The listing builds one solid part. Answer for the finished solid, in the listing's coordinates (mm). Face numbers are marked on the shaded views. Coordinates: 2 decimals unless noted, no trailing zeros. Write each loop counter-clockwise with the first axis right and the second up, starting at its lowest first coordinate (ties: lowest second). Pieces come first, ordered by that corner, then holes.
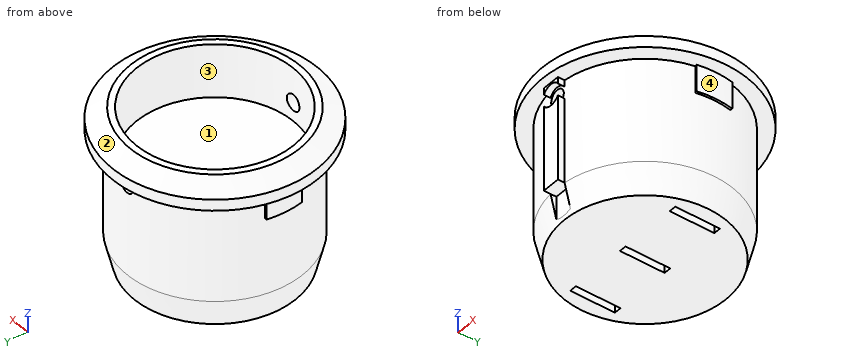
```python
from build123d import *

# Parameters (mm, degrees)
F0_R           = 11.5
F1_DEPTH       = 2.5
F2_R           = 9.85
F3_DEPTH       = 14.8
F4_SIZE2       = 3.2
F4_SIZE        = 0.8
F5_SIZE2       = 1.25
F5_SIZE        = 2
F6_R           = 8.8
F7_DEPTH       = 6
F8_W           = 0.8
F8_H           = 5
F9_DEPTH       = 5
F11_DEPTH      = 11.6
F12_W          = 2
F12_H          = 1.4
F13_DEPTH      = 3.2
F14_R          = 0.9
F15_DEPTH      = 22.0501071022
F17_END_RADIUS = 9.85
F16_R          = 1.2
F17_REACH      = 25.4442196519
F19_DEPTH      = 3


with BuildPart() as f1:
    # F0 (on Top) → F1 (new body)
    with BuildSketch(Plane.XY):
        Circle(F0_R)
    extrude(amount=F1_DEPTH)

    # F2 (on face) → F3 (join)
    with BuildSketch(Plane(origin=(0, 0, 0), x_dir=(1, 0, 0), z_dir=(0, 0, -1))):
        Circle(F2_R)
    extrude(amount=F3_DEPTH)

    # F4
    f4_edges = [f1.edges().sort_by_distance(p)[0] for p in [
        (-9.85, 0, -14.8),
    ]]
    f4_side = f1.faces().sort_by_distance((0, 0, -14.8))[0]
    chamfer(f4_edges, length=F4_SIZE, length2=F4_SIZE2, reference=f4_side)

    # F5
    f5_edges = [f1.edges().sort_by_distance(p)[0] for p in [
        (-11.5, 0, 2.5),
    ]]
    f5_side = f1.faces().sort_by_distance((0, 0, 2.5))[0]
    chamfer(f5_edges, length=F5_SIZE, length2=F5_SIZE2, reference=f5_side)

    # F6 (on face) → F7 (cut)
    with BuildSketch(Plane.XY.offset(2.5)):
        Circle(F6_R)
    extrude(amount=-F7_DEPTH, mode=Mode.SUBTRACT)

    # F8 (on face) → F9 (cut)
    with BuildSketch(Plane(origin=(0, 0, -14.8), x_dir=(1, 0, 0), z_dir=(0, 0, -1))):
        with Locations((-7.1, 0)):
            Rectangle(F8_W, F8_H)
        Rectangle(F8_W, F8_H)
        with Locations((7.1, 0)):
            Rectangle(F8_W, F8_H)
    extrude(amount=-F9_DEPTH, mode=Mode.SUBTRACT)

    # F10 (on face) → F11 (join)
    with BuildSketch(Plane(origin=(0, 0, 0), x_dir=(1, 0, 0), z_dir=(0, 0, -1))):
        with BuildLine():
            Line((-1, 10.5491071022), (-1, 9.7991071022))
            ThreePointArc((-1, 9.7991071022), (0, 9.85), (1, 9.7991071022))
            Line((1, 9.7991071022), (1, 10.5491071022))
            Line((1, 10.5491071022), (-1, 10.5491071022))
        make_face()
    extrude(amount=F11_DEPTH)

    # F12 (on face) → F13 (cut, through all)
    with BuildSketch(Plane(origin=(0, 0, -14.8), x_dir=(1, 0, 0), z_dir=(0, 0, -1))):
        with Locations((0, 9.8491071022)):
            Rectangle(F12_W, F12_H)
    extrude(amount=-F13_DEPTH, mode=Mode.SUBTRACT)

    # F14 (on face) → F15 (cut, through all)
    with BuildSketch(Plane.XZ.offset(10.5491071022)):
        with Locations((0, -1.4)):
            Circle(F14_R)
    extrude(amount=-F15_DEPTH, mode=Mode.SUBTRACT)

    f17_end = (Plane.XY.offset(-5.8) * Cylinder(F17_END_RADIUS, 124.5712732194, mode=Mode.PRIVATE)).faces().sort_by_distance((0, 9.85, -5.8))[0]
    # F16 (on face) → F17 (cut, up to the whole of a round face its end follows)
    with BuildSketch(Plane.XZ.offset(10.5491071022)):
        with Locations((0, -1.4)):
            Circle(F16_R)
    f17_long = extrude(amount=-F17_REACH, mode=Mode.PRIVATE)
    add(split(f17_long, bisect_by=f17_end, keep=Keep.ALL, mode=Mode.PRIVATE).solids().sort_by_distance((0, -10.5491071022, -1.4))[0], mode=Mode.SUBTRACT)

    # F18 (on face) → F19 (join)
    with BuildSketch(Plane(origin=(0, 0, 0), x_dir=(1, 0, 0), z_dir=(0, 0, -1))):
        with BuildLine():
            Line((-9.654950495, 1.9504950495), (-9.9, 2))
            ThreePointArc((-9.9, 2), (-10.1, 0), (-9.9, -2))
            Line((-9.9, -2), (-9.654950495, -1.9504950495))
            ThreePointArc((-9.654950495, -1.9504950495), (-9.85, 0), (-9.654950495, 1.9504950495))
        make_face()
        with BuildLine():
            Line((9.654950495, -1.9504950495), (9.9, -2))
            ThreePointArc((9.9, -2), (10.1, 0), (9.9, 2))
            Line((9.9, 2), (9.654950495, 1.9504950495))
            ThreePointArc((9.654950495, 1.9504950495), (9.85, 0), (9.654950495, -1.9504950495))
        make_face()
    extrude(amount=F19_DEPTH)


solid = f1.part
```
(1) Section B-B, the plane z = -10.5 is taken. Write down the section's boundary in (x, y), plus the area to 3 significant figures.
(2) For a pull along X with two mould halves and no side action, classify the marked faces 1, 2, 3 and 4 as pulls with the +X half, pulls with the -X half, needs draft (parallel to the pull), parting line crosses it, or undercut.
(3) Find the intervals of material crossed by probe 1 along Y at (x, z) = (0, 1); probe 2 along Z at (x, y) = (-5.25, 2.75); probe 3 along X at (y, z) = (-9.1, -1.4), in increasing order.
(4) Each of these flat-tipped pins is pushed along its axis until it touches: pin 1 (1 mm diameter, centred on x = 0, z = -5, fed in from -Y); pin 2 (3 mm diameter, centred on x = 8.5, y = 7.5, fed in from +Z); pin 3 (5.5 mm diameter, centred on y = 0, z = -11.5, fed in from +X); pin 4 (1.1 mm diameter, centred on x = 0, z = -1.4, fed in from +Y). Where does it stop, or does it pass through?
(5) Section A-A, the plane x = 0 is taken. State how many separate pieces and enclosed holes the cut face has, plus the area to 3 significant figures.
(6) Section C-C, the plane z = -1.4 is taken. Write down the section's boundary in (x, y), plus the area to 3 significant figures.
Solution:
1. outline: (-1, -10.55) - (1, -10.55) - (1, -9.8) arc R9.85 ccw (long way) to (-1, -9.8) - close; hole (-7.5, -2.5) - (-6.7, -2.5) - (-6.7, 2.5) - (-7.5, 2.5) - close; hole (-0.4, -2.5) - (0.4, -2.5) - (0.4, 2.5) - (-0.4, 2.5) - close; hole (6.7, -2.5) - (7.5, -2.5) - (7.5, 2.5) - (6.7, 2.5) - close
1. area: 294 mm2
2. face 1: undercut
2. face 2: parting line crosses it
2. face 3: undercut
2. face 4: pulls with the +X half
3. probe 1: y = -11.5 to -8.8, 8.8 to 11.5
3. probe 2: z = -14.8 to -3.5
3. probe 3: x = -3.77 to -0.9, 0.9 to 3.77
4. pin 1: stops at y = -10.55
4. pin 2: stops at z = 2.29
4. pin 3: stops at x = 9.85
4. pin 4: passes through
5. separate pieces: 3
5. enclosed holes: 0
5. area: 215 mm2
6. outline: (-9.9, -2) - (-9.65, -1.95) arc R9.85 ccw to (-0.9, -9.81) - (-0.9, -8.75) arc R8.8 cw to (-0.9, 8.75) - (-0.9, 9.81) arc R9.85 ccw to (-9.65, 1.95) - (-9.9, 2) arc R10.1 ccw to start; (0.9, -9.81) arc R9.85 ccw to (9.65, -1.95) - (9.9, -2) arc R10.1 ccw to (9.9, 2) - (9.65, 1.95) arc R9.85 ccw to (0.9, 9.81) - (0.9, 8.75) arc R8.8 cw to (0.9, -8.75) - close
6. area: 59.7 mm2
